Verification items for this drawing (mm, ordinates from the low corner). A direction names the side the tool comes from. Coordinates: 2 decimals unless noted, no trailing zeros. Order: outer loops, then holes, each group sorted by start corner. A loop starts at its lowest first (then second) coordinate and runs counter-clockwise, first axis right, second up. Notation, with made-up numbers: M -21,83 L 4,83 A24 ccw 4,120 Z; hole C 39,71.25 d3. An arc over 180 degrees is marked long. One line per item, written item: value. Start each with the question number.
1) Go/stop test with a flat-tipped pin: P1, Ø6.5, axis at x = 25, z = 8.5, coming from the -Y side. Record where the tip stops, or that it passes through.
2) Sectioned sample at B-B, the plane x = 36. Enter the section's corners in (y, z).
3) Sectioned sample at D-D, the plane x = 25. Enter the section's corners in (y, z).
4) Sectioned sample at C-C, the plane y = 10. Enter the section's corners in (x, z).
5) Sectioned sample at A-A, the plane z = 8.5. Enter the section's corners in (x, y).
6) Draft check along X on the marked faces 3, 4 and 5. Enter one of: pulls with the +X half, pulls with the -X half, needs draft (parallel to the pull), parting line crosses it, or undercut.
7) Access from +Z, -Z, +X, -X, +Y, -Y to the whole of each face (thin tool, end or side, straight path). Record for the marked faces 1 and 2.
8) Thickness scan on L1, parallel to Z at x = 25, y = 29.85; L2, parallel to X at y = 12.5, z = 15; L3, parallel to Y at x = 22, z = 15.5. Record the ranges inside material, lowest first. Write a range as from..to.
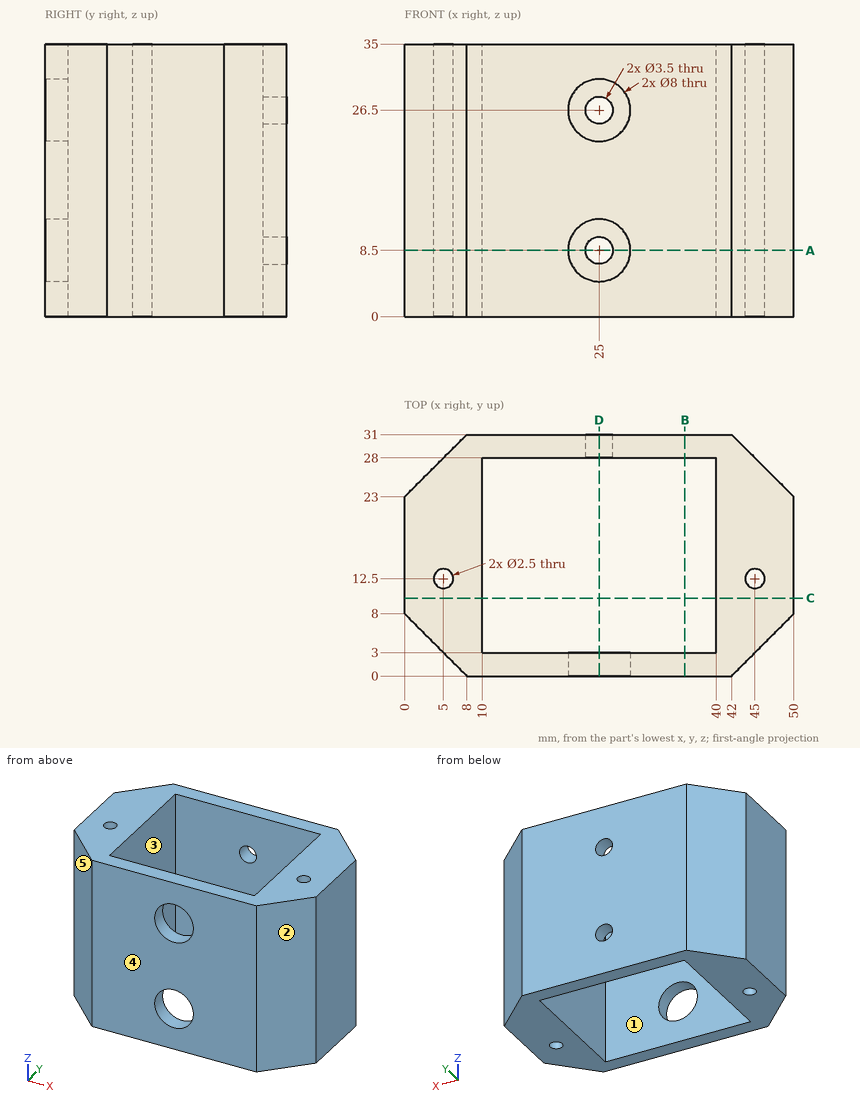
Final values:
1. P1: stops at y = 28
2. outline: M 0,0 L 3,0 L 3,35 L 0,35 Z; M 28,0 L 31,0 L 31,35 L 28,35 Z
3. outline: M 0,0 L 3,0 L 3,4.5 L 0,4.5 Z; M 0,12.5 L 3,12.5 L 3,22.5 L 0,22.5 Z; M 0,30.5 L 3,30.5 L 3,35 L 0,35 Z; M 28,0 L 31,0 L 31,6.75 L 28,6.75 Z; M 28,10.25 L 31,10.25 L 31,24.75 L 28,24.75 Z; M 28,28.25 L 31,28.25 L 31,35 L 28,35 Z
4. outline: M 0,0 L 10,0 L 10,35 L 0,35 Z; M 40,0 L 50,0 L 50,35 L 40,35 Z
5. outline: M 0,8 L 8,0 L 21,0 L 21,3 L 10,3 L 10,28 L 23.25,28 L 23.25,31 L 8,31 L 0,23 Z; M 26.75,28 L 40,28 L 40,3 L 29,3 L 29,0 L 42,0 L 50,8 L 50,23 L 42,31 L 26.75,31 Z; hole C 5,12.5 d2.5; hole C 45,12.5 d2.5
6. face 3: undercut
6. face 4: needs draft
6. face 5: pulls with the -X half
7. face 1: +Z, -Z
7. face 2: +Z, -Z, +X, -Y
8. L1: z = 0..6.75, 10.25..24.75, 28.25..35
8. L2: x = 0..3.75, 6.25..10, 40..43.75, 46.25..50
8. L3: y = 0..3, 28..31
